Input: part model. Units: mm. Frame: model coordinates. Face numbers are marked on the shaded views. A direction names the side the tool comes from. Give positions to 0.01 mm unless a question says otherwise; leave off trailing zeros. Write each loop counter-clockwise with the first axis right and the second up, starting at its lowest first coordinate (ties: lowest second). Pieces come first, ordered by that corner, then holes. Notation, with made-up numbers: M 51,4.25 L 99,4.25 A31 cw 99,37.25 Z; hole C 12.25,37.25 d10. An arc over 180 degrees is marked long. Use CSV: the item, a comma, the result in double quotes. Start each with the question number.
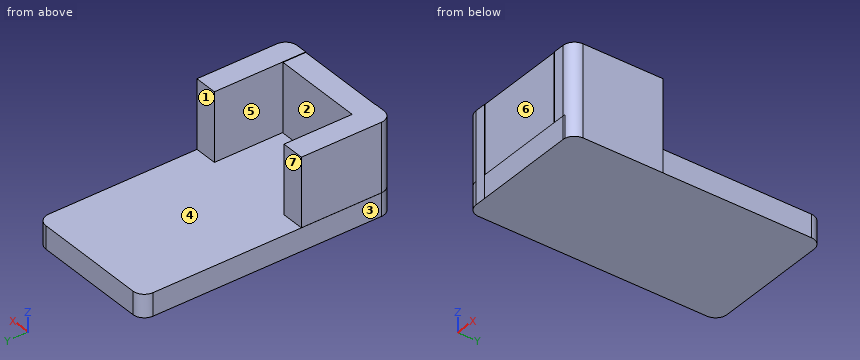
from build123d import *

# Parameters (mm, degrees)
F1_DEPTH = 12.7
F3_DEPTH = 50.8
F4_W     = 50.8
F4_H     = 12.7
F5_DEPTH = 50.8


with BuildPart() as f1:
    # F0 (on Top) → F1 (new body)
    with BuildSketch(Plane.XY):
        with BuildLine():
            ThreePointArc((38.1, 63.5), (36.240128, 67.990128), (31.75, 69.85))
            Line((31.75, 69.85), (-31.75, 69.85))
            ThreePointArc((-31.75, 69.85), (-36.240128, 67.990128), (-38.1, 63.5))
            Line((-38.1, 63.5), (-38.1, -63.5))
            ThreePointArc((-38.1, -63.5), (-36.240128, -67.990128), (-31.75, -69.85))
            Line((-31.75, -69.85), (31.75, -69.85))
            ThreePointArc((31.75, -69.85), (36.240128, -67.990128), (38.1, -63.5))
            Line((38.1, -63.5), (38.1, 63.5))
        make_face()
    extrude(amount=F1_DEPTH)

    # F2 (on Top) → F3 (join)
    with BuildSketch(Plane.XY):
        with BuildLine():
            Line((-25.359782, -19.050035), (-38.059782, -19.050035))
            Line((-38.059782, -19.050035), (-38.059782, -63.500035))
            ThreePointArc((-38.059782, -63.500035), (-36.19991, -67.990163), (-31.709782, -69.850035))
            Line((-31.709782, -69.850035), (-25.359782, -69.850035))
            Line((-25.359782, -69.850035), (-25.359782, -19.050035))
        make_face()
        with BuildLine():
            Line((38.140218, -19.040707), (25.440218, -19.040707))
            Line((25.440218, -19.040707), (25.440218, -69.840707))
            Line((25.440218, -69.840707), (31.790218, -69.840707))
            ThreePointArc((31.790218, -69.840707), (36.280346, -67.980835), (38.140218, -63.490707))
            Line((38.140218, -63.490707), (38.140218, -19.040707))
        make_face()
    extrude(amount=F3_DEPTH)

    # F4 (on Top) → F5 (join)
    with BuildSketch(Plane.XY):
        with Locations((-0.266136, -63.306491)):
            Rectangle(F4_W, F4_H)
    extrude(amount=F5_DEPTH)


solid = f1.part
Q1. Pull-direction query (X, two-part tool) for the marked faces 1, 2, 3 and 4; classes: released by +X, released by -X, zero draft, split by the parting line, or undercut.
Q2. Section A-A, the plane z = 36. Return the cut outline in (x, y).
Q3. Set-up query: the marked faces 5, 6 and 7. Return all of +Z, -Z, +X, -X, +Y, -Y with unobstructed straight access to the full face (end or side cutting, diameter ignored); none if empty.
Q4. First-contact query: pin 1 Ø14 at (y, z) = (33, 7) entering from +X; pin 2 Ø10 at (x, z) = (-32.5, 35) entering from +Y; pin 3 Ø7 at (x, z) = (29, 30) entering from -Y. Flat tips, straight axial feed; report the tip coordinate or a pass-through.
Q5. Material intervals for L1, parallel to Y at x = 27, z = 31; L2, parallel to X at y = -60.5, z = 48; L3, parallel to Y at x = -26, z = 48, sorted ascending. Write a range as [from, to].
Q6. Section C-C, the plane y = -43. Return the cut outline in (x, z).
Q7. Section D-D, the plane x = -17.5. Return the cut outline in (y, z), and give its area (3 significant figures).
Check result:
1,face 1,"zero draft"
1,face 2,"undercut"
1,face 3,"released by -X"
1,face 4,"undercut"
2,outline,"M -38.06,-63.5 A6.35 ccw -31.71,-69.85 L -25.36,-69.85 L -25.36,-69.66 L 25.13,-69.66 L 25.13,-56.96 L -25.36,-56.96 L -25.36,-19.05 L -38.06,-19.05 Z; M 25.44,-69.84 L 31.79,-69.84 A6.35 ccw 38.14,-63.49 L 38.14,-19.04 L 25.44,-19.04 Z"
3,face 5,"+Z, +Y, -Y"
3,face 6,"+Z, -Y"
3,face 7,"+Z, +X, -X, +Y"
4,pin 1,"stops at x = 38.1"
4,pin 2,"stops at y = -19.05"
4,pin 3,"stops at y = -69.84"
5,L1,"y = [-69.84, -19.04]"
5,L2,"x = [-38.06, 25.13], [25.44, 38.14]"
5,L3,"y = [-69.85, -19.05]"
6,outline,"M -38.1,0 L 38.14,0 L 38.14,50.8 L 25.44,50.8 L 25.44,12.7 L -25.36,12.7 L -25.36,50.8 L -38.06,50.8 L -38.06,12.7 L -38.1,12.7 Z"
7,outline,"M -69.85,0 L 69.85,0 L 69.85,12.7 L -56.96,12.7 L -56.96,50.8 L -69.66,50.8 L -69.66,12.7 L -69.85,12.7 Z"
7,area,"2,260 mm²"
